Geometry: final body of the model. Coordinates: model frame, mm. Face numbers are marked on the shaded views. A direction names the side the tool comes from. Give positions to 0.01 mm unless a question says otherwise; leave off trailing zeros. Write each loop counter-clockwise with the first axis right and the second up, starting at its lowest first coordinate (ties: lowest second). Pieces come first, ordered by that corner, then holes.
Q1. Cut plane C-C on x = 6.35. Return the cut outline in (y, z).
Q2. Line query: L1, parallel to X at y = 5.75, z = 0; L2, parallel to Z at x = -40, y = 5; L3, parallel to X at y = 0.75, z = 2. Output: solid intervals per line, ascending.
Q3. Pin query (flat end, axial travel): pin 1 (1.8 mm diameter, centred on x = -43.5, y = 4, fed in from -Z); pin 2 (4 mm diameter, centred on x = -57.15, z = 0, fed in from +Y); pin 3 (1 mm diameter, centred on y = 3, z = -10, fed in from +X); pin 4 (1.8 mm diameter, centred on x = -34.5, y = 4.5, fed in from +Z). Return the tip coordinate at first contact, or that it passes through.
Q4. Reachability of the marked faces 4, 5 and 6 from +Z, -Z, +X, -X, +Y, -Y: full face, straight path, thin tool, end or side. Return the list, or none.
Q5. Cut plane A-A on z = -11.5. Return the cut outline in (x, y), plus the area to 3 significant figures.
Q6. Cut plane B-B on y = 1.25. Count the separate pieces of the cut face and the enclosed holes in it, plus the area to 3 significant figures.
Q7. Draft query along Z for the marked faces 1, 2 and 3. Return one class per face: pulls with the +Z half, pulls with the -Z half, needs draft (parallel to the pull), parting line crosses it, or undercut.
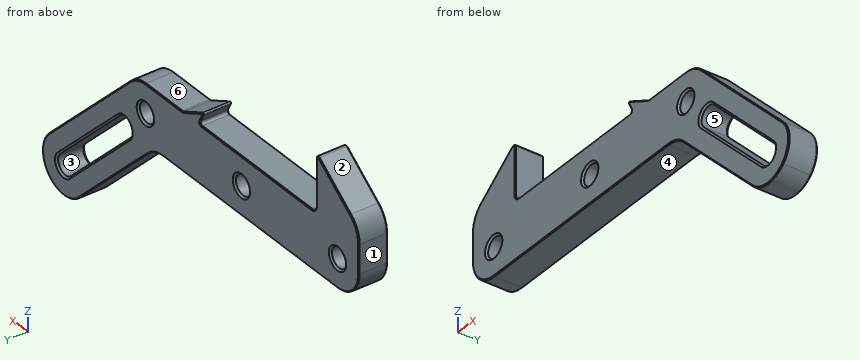
```python
from build123d import *

# Parameters (mm, degrees)
SKETCH1_R           = 2.1828125
BOSS_EXTRUDE1_DEPTH = 6.35
CHAMFER2_SIZE       = 0.396875
CHAMFER3_SIZE       = 0.1984375


with BuildPart() as part:
    # Sketch1 → Boss-Extrude1 (new body)
    with BuildSketch(Plane(origin=(0, 0, 0), x_dir=(1, 0, 0), z_dir=(0, 1, 0))):
        with BuildLine():
            Line((-50.8, -7.62), (-50.8, -18.034))
            ThreePointArc((-50.8, -18.034), (-51.080815493, -18.488369013), (-51.6128, -18.4404))
            Line((-51.6128, -18.4404), (-60.9601016, -11.4299238))
            ThreePointArc((-60.9601016, -11.4299238), (-62.829639478, -9.189819739), (-63.5, -6.350127))
            Line((-63.5, -6.350127), (-63.5, 0.000254))
            ThreePointArc((-63.5, 0.000254), (-61.640202455, 4.490202455), (-57.150254, 6.35))
            Line((-57.150254, 6.35), (-5.260407032, 6.35))
            ThreePointArc((-5.260407032, 6.35), (-2.830464438, 6.833345634), (-0.770458576, 8.209797545))
            Line((-0.770458576, 8.209797545), (19.820563787, 28.800819908))
            ThreePointArc((19.820563787, 28.800819908), (24.310512242, 30.660617452), (28.800819908, 28.800460698))
            ThreePointArc((28.800819908, 28.800460698), (30.660617452, 24.310512242), (28.800819908, 19.820563787))
            Line((28.800819908, 19.820563787), (4.490053666, -4.490202455))
            ThreePointArc((4.490053666, -4.490202455), (2.430047804, -5.866654366), (0.00010521, -6.35))
            Line((0.00010521, -6.35), (-10.812693667, -6.35))
            ThreePointArc((-10.812693667, -6.35), (-11.104479877, -6.383973783), (-11.380654934, -6.484077467))
            Line((-11.380654934, -6.484077467), (-16.780946479, -9.18422324))
            ThreePointArc((-16.780946479, -9.18422324), (-17.074143855, -9.136643856), (-17.121723239, -8.84344648))
            Line((-17.121723239, -8.84344648), (-16.242592252, -7.085184507))
            ThreePointArc((-16.242592252, -7.085184507), (-16.264830655, -6.590928595), (-16.696961265, -6.35))
            Line((-16.696961265, -6.35), (-49.53, -6.35))
            ThreePointArc((-49.53, -6.35), (-50.428025612, -6.721974388), (-50.8, -7.62))
        make_face()
        Circle(SKETCH1_R, mode=Mode.SUBTRACT)
        with Locations((-57.150254, 0.000254)):
            Circle(SKETCH1_R, mode=Mode.SUBTRACT)
        with Locations((-28.574999999, 0.000254)):
            Circle(SKETCH1_R, mode=Mode.SUBTRACT)
        with BuildLine():
            Line((4.806518479, 7.893481521), (22.767030721, 25.853993763))
            ThreePointArc((22.767030721, 25.853993763), (25.853993763, 25.853993763), (25.853993763, 22.767030721))
            Line((25.853993763, 22.767030721), (7.893481521, 4.806518479))
            ThreePointArc((7.893481521, 4.806518479), (4.806518479, 4.806518479), (4.806518479, 7.893481521))
        make_face(mode=Mode.SUBTRACT)
    extrude(amount=BOSS_EXTRUDE1_DEPTH)

    # Chamfer2
    chamfer2_edges = [part.edges().sort_by_distance(p)[0] for p in [
        (-2.1828125, 0, 0),
        (-2.1828125, 6.35, 0),
        (4.806518479, 0, -4.806518479),
        (16.873737642, 0, -13.7867746),
        (25.853993763, 0, -25.853993763),
        (13.7867746, 0, -16.873737642),
        (4.806518479, 6.35, -4.806518479),
        (16.873737642, 6.35, -13.7867746),
        (25.853993763, 6.35, -25.853993763),
        (13.7867746, 6.35, -16.873737642),
        (-59.3330665, 0, -0.000254),
        (-59.3330665, 6.35, -0.000254),
        (-30.757812499, 0, -0.000254),
        (-30.757812499, 6.35, -0.000254),
    ]]
    chamfer(chamfer2_edges, length=CHAMFER2_SIZE)

    # Chamfer3
    chamfer3_edges = [part.edges().sort_by_distance(p)[0] for p in [
        (-2.830464438, 6.35, -6.833345634),
        (-31.205330516, 6.35, -6.35),
        (-61.640202455, 6.35, -4.490202455),
        (24.310766246, 0, -30.660617447),
        (30.660617452, 0, -24.310512242),
        (16.645436787, 0, -7.665180666),
        (2.430047804, 0, 5.866654366),
        (-5.406294229, 0, 6.35),
        (-11.104479877, 0, 6.383973783),
        (-14.080800707, 0, 7.834150354),
        (-17.074143855, 0, 9.136643856),
        (-16.682157746, 0, 7.964315493),
        (-16.264830655, 0, 6.590928595),
        (-63.5, 6.35, 3.1749365),
        (-33.113480633, 0, 6.35),
        (-50.428025612, 0, 6.721974388),
        (-50.8, 0, 12.827),
        (-51.080815493, 0, 18.488369013),
        (-56.2864508, 0, 14.9351619),
        (-62.829639478, 0, 9.189819739),
        (-63.5, 0, 3.1749365),
        (-61.640202455, 0, -4.490202455),
        (-31.205330516, 0, -6.35),
        (-2.830464438, 0, -6.833345634),
        (-62.829639478, 6.35, 9.189819739),
        (9.525052605, 0, -18.505308726),
        (24.310766246, 0, -30.660617447),
        (-56.2864508, 6.35, 14.9351619),
        (-51.080815493, 6.35, 18.488369013),
        (-50.8, 6.35, 12.827),
        (-50.428025612, 6.35, 6.721974388),
        (-33.113480633, 6.35, 6.35),
        (24.310766246, 6.35, -30.660617447),
        (-16.264830655, 6.35, 6.590928595),
        (-16.682157746, 6.35, 7.964315493),
        (-17.074143855, 6.35, 9.136643856),
        (-14.080800707, 6.35, 7.834150354),
        (-11.104479877, 6.35, 6.383973783),
        (-5.406294229, 6.35, 6.35),
        (2.430047804, 6.35, 5.866654366),
        (16.645436787, 6.35, -7.665180666),
        (30.660617452, 6.35, -24.310512242),
        (24.310766246, 6.35, -30.660617447),
        (9.525052605, 6.35, -18.505308726),
    ]]
    chamfer(chamfer3_edges, length=CHAMFER3_SIZE)


solid = part.part
```
Data:
1. outline: (0, -15.05) - (0.2, -15.33) - (6.15, -15.33) - (6.35, -15.05) - (6.35, -10) - (5.95, -9.44) - (0.4, -9.44) - (0, -10) - close; (0, -3.77) - (0.4, -4.17) - (5.95, -4.17) - (6.35, -3.77) - (6.35, 2.35) - (6.15, 2.63) - (0.2, 2.63) - (0, 2.35) - close
2. L1: x = -63.5 to -59.33, -54.97 to -30.76, -26.39 to -2.18, 2.18 to 8.98
2. L2: z = -6.35 to 6.35
2. L3: x = -63.5 to -58.02, -56.28 to -29.45, -27.7 to -0.87, 0.87 to 6.98
3. pin 1: stops at z = -6.35
3. pin 2: passes through
3. pin 3: stops at x = 19.48
3. pin 4: stops at z = 6.35
4. face 4: -Z, -X, +Y, -Y
4. face 5: +Y, -Y
4. face 6: +Z, +X, +Y, -Y
5. outline: (2.52, 0.2) - (2.8, 0) - (7.85, 0) - (8.41, 0.4) - (8.41, 5.95) - (7.85, 6.35) - (2.8, 6.35) - (2.52, 6.15) - close; (14.59, 0.4) - (15.15, 0) - (20.2, 0) - (20.48, 0.2) - (20.48, 6.15) - (20.2, 6.35) - (15.15, 6.35) - (14.59, 5.95) - close
5. area: 74.3 mm2
6. separate pieces: 1
6. enclosed holes: 4
6. area: 1,230 mm2
7. face 1: needs draft
7. face 2: pulls with the +Z half
7. face 3: undercut
